Autodesk Inventor part; units mm, degrees
ref_plane "YZ Plane" through (0, 0, 0) normal (1, 0, 0) x (0, 1, 0)
ref_plane "XZ Plane" through (0, 0, 0) normal (0, 1, 0) x (-1, 0, 0)
ref_plane "XY Plane" through (0, 0, 0) normal (0, 0, 1) x (1, 0, 0)
sketch "Sketch1" plane through (0, 0, 0) normal (0, 1, 0) x (-1, 0, 0)
  line L0 (3.9, -2.8393) -> (3.9, 2.8393)
  line L1 (2.8393, 3.9) -> (-2.8393, 3.9)
  line L2 (-2.8393, -3.9) -> (2.8393, -3.9)
  line L3 (8.5707, 3.2957) -> (10, 4.725)
  line L4 (8.5707, -3.2957) -> (10, -4.725)
  line L5 (8.4, 3.3664) -> (8.4, 6)
  line L6 (8.4, 6) -> (7.0607, 6)
  line L7 (10, 9) -> (10, 4.725)
  line L8 (10, -4.725) -> (10, -9)
  line L9 (3.9, 2.8393) -> (7.0607, 6)
  line L10 (3.2957, 8.5707) -> (4.725, 10)
  line L11 (3.3664, 8.4) -> (6, 8.4)
  line L12 (6, 8.4) -> (6, 7.0607)
  line L13 (2.8393, 3.9) -> (6, 7.0607)
  line L14 (3.9, 0) -> (8.4, 0)
  line L15 (8.4, -3.3664) -> (8.4, -6)
  line L16 (8.4, -6) -> (7.0607, -6)
  line L17 (3.9, -2.8393) -> (7.0607, -6)
  line L18 (3.2957, -8.5707) -> (4.725, -10)
  line L19 (3.3664, -8.4) -> (6, -8.4)
  line L20 (6, -8.4) -> (6, -7.0607)
  line L21 (2.8393, -3.9) -> (6, -7.0607)
  line L22 (-3.9, -2.8393) -> (-3.9, 2.8393)
  line L23 (-8.5707, 3.2957) -> (-10, 4.725)
  line L24 (-8.5707, -3.2957) -> (-10, -4.725)
  line L25 (-8.4, 3.3664) -> (-8.4, 6)
  line L26 (-8.4, 6) -> (-7.0607, 6)
  line L27 (-10, 9) -> (-10, 4.725)
  line L28 (-10, -4.725) -> (-10, -9)
  line L29 (-3.9, 2.8393) -> (-7.0607, 6)
  line L30 (-3.2957, 8.5707) -> (-4.725, 10)
  line L31 (-3.3664, 8.4) -> (-6, 8.4)
  line L32 (-6, 8.4) -> (-6, 7.0607)
  line L33 (-2.8393, 3.9) -> (-6, 7.0607)
  line L34 (-3.9, -2.8393) -> (-7.0607, -6)
  line L35 (-8.4, -6) -> (-7.0607, -6)
  line L36 (-8.4, -3.3664) -> (-8.4, -6)
  line L37 (-2.8393, -3.9) -> (-6, -7.0607)
  line L38 (-6, -8.4) -> (-6, -7.0607)
  line L39 (-3.3664, -8.4) -> (-6, -8.4)
  line L40 (-3.2957, -8.5707) -> (-4.725, -10)
  line L41 (-9, 10) -> (-4.725, 10)
  line L42 (4.725, 10) -> (9, 10)
  line L43 (9, -10) -> (4.725, -10)
  line L44 (-4.725, -10) -> (-9, -10)
  circle A0 centre (0, 0) radius 2.1
  arc A1 (10, 9) -> (9, 10) centre (9, 9) ccw
  arc A2 (9, -10) -> (10, -9) centre (9, -9) ccw
  arc A3 (-10, -9) -> (-9, -10) centre (-9, -9) ccw
  arc A4 (-9, 10) -> (-10, 9) centre (-9, 9) ccw
  arc A5 (8.4, 3.3664) -> (8.5707, 3.2957) centre (8.5, 3.3664) ccw
  arc A6 (3.2957, 8.5707) -> (3.3664, 8.4) centre (3.3664, 8.5) ccw
  arc A7 (8.5707, -3.2957) -> (8.4, -3.3664) centre (8.5, -3.3664) ccw
  arc A8 (3.3664, -8.4) -> (3.2957, -8.5707) centre (3.3664, -8.5) ccw
  arc A9 (-3.2957, -8.5707) -> (-3.3664, -8.4) centre (-3.3664, -8.5) ccw
  arc A10 (-8.4, -3.3664) -> (-8.5707, -3.2957) centre (-8.5, -3.3664) ccw
  arc A11 (-8.5707, 3.2957) -> (-8.4, 3.3664) centre (-8.5, 3.3664) ccw
  arc A12 (-3.3664, 8.4) -> (-3.2957, 8.5707) centre (-3.3664, 8.5) ccw
  dimension "d11" = 1
extrude "Extrusion1" add sketch "Sketch1" along normal blind 280
properties part number "VSLOT20x20x280"
Source: CAD feature listing. Evaluate the final solid. Frame: model axes, mm. A direction names the side the tool comes from. Round coordinates to 2 decimals unless told otherwise and drop trailing zeros. Answer as a JSON object with one key per item and string values. Group by question number.
Q1. Mould query, pull axis Z, two halves, no side actions, for faces 1 (the flat face through (3.9, 138, 0)), 2 (the flat face through (-7, 138, 10)), 3 (the flat face through (-3.9, 138, 0)), 4 (the flat face through (-10, 138, -7)). Classes: pulls with the +Z half, pulls with the -Z half, needs draft (parallel to the pull), parting line crosses it, or undercut.
Q2. Ray query, line 1 (Z direction, x = 0, y = 65.5); line 2 (X direction, y = 53, z = -5); line 3 (X direction, y = 226, z = -8.5). Return the intervals inside material, ascending. Write a range as from..to.
Q3. Access query for faces 5 (the flat face through (0, 138, 3.9)), 6 (the flat face through (0, 138, -3.9)), 7 (the flat face through (-7, 138, -10)). Directions: +Z, -Z, +X, -X, +Y, -Y. A direction counts if a zero-diameter tool reaches every point of the face in a straight line with its end or side. Return the directions, or none.
Q4. Contact query for flat-ended pins moving along their axis: P1, Ø4.5, axis at y = 75.5, z = 0.5, coming from the +X side; P2, Ø5, axis at y = 94, z = -1, coming from the -X side (3 decimals); P3, Ø6, axis at x = 1.5, y = 73, coming from the -Z side (3 decimals). Output: stop coordinate, or through.
Completed:
{
 "1": {"face 1": "undercut", "face 2": "pulls with the +Z half", "face 3": "undercut", "face 4": "needs draft"},
 "2": {"line 1": "-3.9..-2.1, 2.1..3.9", "line 2": "-10..-8.4, -6.06..-3.94, 3.94..6.06, 8.4..10", "line 3": "-10..-3.27, 3.27..10"},
 "3": {"face 5": "+Z, +Y, -Y", "face 6": "-Z, +Y, -Y", "face 7": "-Z, +X, -X, +Y, -Y"},
 "4": {"P1": "x = 3.9", "P2": "x = -8.775", "P3": "z = -9.775"}
}
